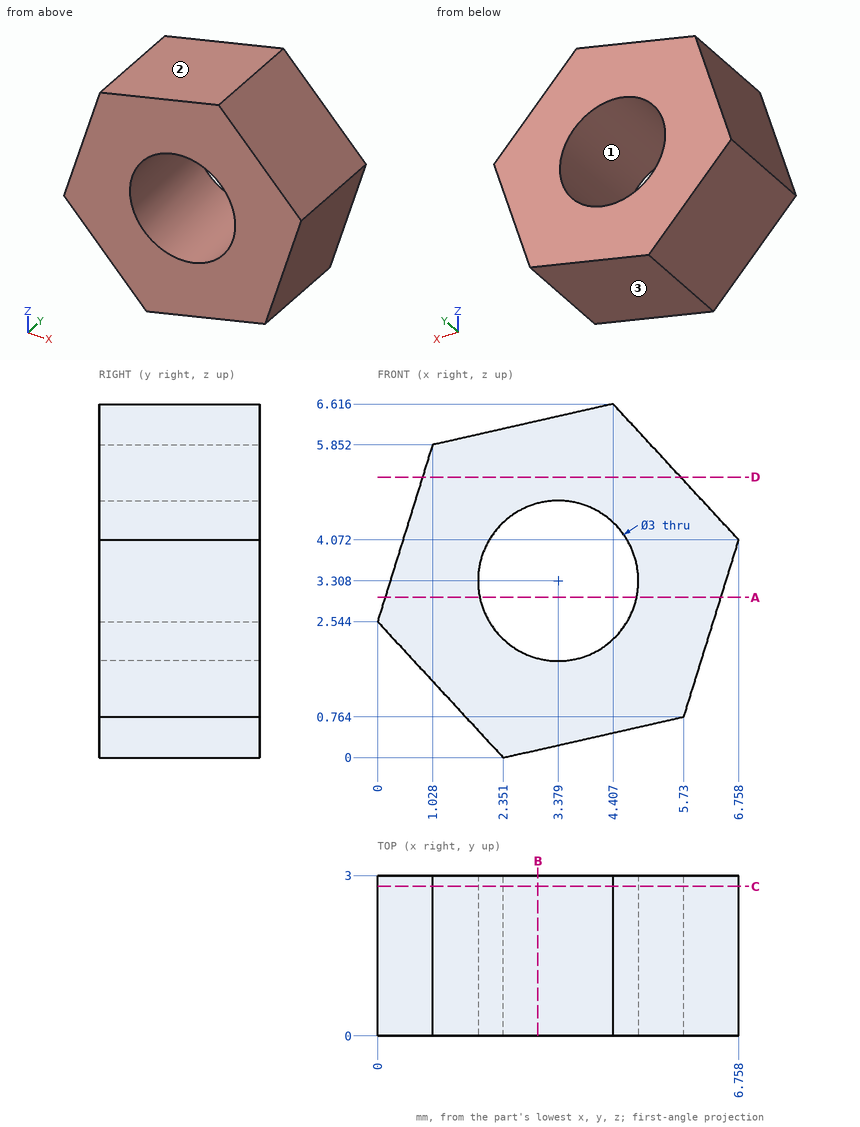
Here's the drawing with two shaded views (mm, measured from the low corner). I have some questions. Give positions to 0.01 mm unless a question says otherwise; leave off trailing zeros. Order: outer loops, then holes, each group sorted by start corner. A loop starts at its lowest first (then second) coordinate and runs counter-clockwise, first axis right, second up. Notation, with made-up numbers: M 43,-21.75 L 76,-21.75 A15 cw 76,-2.75 Z; hole C 41.25,69.5 d6. An arc over 180 degrees is marked long. Answer as a JSON object with one key per item and string values. Group by question number.
1) We'd pull the mould along X, two halves only. Please class the marked faces 1, 2 and 3: pulls with the +X half, pulls with the -X half, needs draft (parallel to the pull), parting line crosses it, or undercut.
2) Suppose I cut it at B-B, the plane x = 3. Write out the boundary of the cut face in (y, z).
3) Please list where these lines run through material, in increasing order: L1, parallel to X at y = 0.45, z = 3.75 (1 decimal); L2, parallel to Z at x = 2.5, y = 2.8 (1 decimal); L3, parallel to X at y = 1.65, z = 3 (1 decimal). Write a range as [from, to].
4) I'm going to push a flat-ended pin straight in: pin 1 Ø1.5 at (y, z) = (1.5, 1.5) entering from -X. Where does the tip first touch, or does it pass through?
5) Suppose I cut it at A-A, the plane z = 3. Write out the boundary of the cut face in (x, y) (1 decimal).
6) Suppose I cut it at D-D, the plane z = 5.25. Write out the boundary of the cut face in (x, y), plus the area to 3 significant figures.
7) Suppose I cut it at C-C, the plane y = 2.8. Write out the boundary of the cut face in (x, z), plus the area to 3 significant figures.
Results found:
{
 "1": {"face 1": "undercut", "face 2": "pulls with the -X half", "face 3": "pulls with the +X half"},
 "2": {"outline": "M 0,0.15 L 3,0.15 L 3,1.86 L 0,1.86 Z; M 0,4.76 L 3,4.76 L 3,6.3 L 0,6.3 Z"},
 "3": {"L1": "[0.4, 1.9], [4.8, 6.7]", "L2": "[0, 2.1], [4.5, 6.2]", "L3": "[0.1, 1.9], [4.8, 6.4]"},
 "4": {"pin 1": "x = 0.27"},
 "5": {"outline": "M 0.1,0 L 1.9,0 L 1.9,3 L 0.1,3 Z; M 4.8,0 L 6.4,0 L 6.4,3 L 4.8,3 Z"},
 "6": {"outline": "M 0.84,0 L 5.67,0 L 5.67,3 L 0.84,3 Z", "area": "14.5 mm²"},
 "7": {"outline": "M 0,2.54 L 2.35,0 L 5.73,0.76 L 6.76,4.07 L 4.41,6.62 L 1.03,5.85 Z; hole C 3.38,3.31 d3", "area": "24.1 mm²"}
}
